Source: CAD feature listing. Evaluate the final solid. Frame: model axes, mm. A direction names the side the tool comes from. Coordinates: 2 decimals unless noted, no trailing zeros. Order: outer loops, then holes, each group sorted by start corner. A loop starts at its lowest first (then second) coordinate and runs counter-clockwise, first axis right, second up. Notation, with made-up numbers: (8.5, 30.25) -> (18.5, 30.25) arc R24 cw to (18.5, 58.25) -> close; hole circle Ø11 at (8, 72.5). An arc over 180 degrees is marked (long way). Write item = value, one per line. Start each with the question number.
Item 1: Contact query for flat-ended pins moving along their axis: pin 1 (1.5 mm diameter, centred on y = -428.5, z = 632, fed in from -X); pin 2 (1.5 mm diameter, centred on x = 108, y = -996.5, fed in from +Z); pin 3 (10 mm diameter, centred on x = 606, z = 1258, fed in from -Y). Output: stop coordinate, or through.
Item 2: Section query A-A (x = 641). Output: boundary loops of the cut face in (y, z).
Item 3: Section query B-B (y = -1621.5). Output: boundary loops of the cut face in (x, z), then the cut area to 3 significant figures.
Item 4: Section query D-D (x = 494.5). Output: boundary loops of the cut face in (y, z), then the cut area to 3 significant figures.
Item 5: Set-up query: faces 1 (the flat face through (351, -1102, 0)), 2 (the flat face through (509, -2033, 273.05)), 3 (the flat face through (272, -1796, 546.1)). Return all of +Z, -Z, +X, -X, +Y, -Y with unobstructed straight access to the full face (end or side cutting, diameter ignored); none if empty.
Item 6: Section query C-C (z = 621.5). Output: boundary loops of the cut face in (x, y), then the cut area to 3 significant figures.
Item 7: Ray query, line 1 along Z through (x, y) = (220, -876.5); line 2 along Z through (x, y) = (356, -1162); line 3 along Y through (x, z) = (382, 1186). Return the intervals inside material, ascending. Write a range as [from, to].
```python
from build123d import *

# Parameters (mm, degrees)
F0_W      = 711.2
F0_H      = 2235.2
F1_DEPTH  = 273.05
F3_DEPTH  = 273.05
F4_W      = 711.2
F4_H      = 1524
F5_DEPTH  = 273.05
F6_W      = 711.2
F6_H      = 1143
F7_DEPTH  = 273.05
F8_W      = 711.2
F8_H      = 762
F9_DEPTH  = 273.05
F10_W     = 711.2
F10_H     = 381
F11_DEPTH = 273.05


with BuildPart() as f1:
    # F0 (on Top) → F1 (new body)
    with BuildSketch(Plane.XY):
        with Locations((355.6, -1117.6)):
            Rectangle(F0_W, F0_H)
    extrude(amount=F1_DEPTH)

    # F2 (on face) → F3 (join)
    with BuildSketch(Plane.XY.offset(273.05)):
        Polygon((0, 0), (0, -2235.2), (711.2, -1524), (711.2, 0), align=None)
    extrude(amount=F3_DEPTH)

    # F4 (on face) → F5 (join)
    with BuildSketch(Plane.XY.offset(546.1)):
        with Locations((355.6, -762)):
            Rectangle(F4_W, F4_H)
    extrude(amount=F5_DEPTH)

    # F6 (on face) → F7 (join)
    with BuildSketch(Plane.XY.offset(819.15)):
        with Locations((355.6, -571.5)):
            Rectangle(F6_W, F6_H)
    extrude(amount=F7_DEPTH)

    # F8 (on face) → F9 (join)
    with BuildSketch(Plane.XY.offset(1092.2)):
        with Locations((355.6, -381)):
            Rectangle(F8_W, F8_H)
    extrude(amount=F9_DEPTH)

    # F10 (on face) → F11 (join)
    with BuildSketch(Plane.XY.offset(1365.25)):
        with Locations((355.6, -190.5)):
            Rectangle(F10_W, F10_H)
    extrude(amount=F11_DEPTH)


solid = f1.part
```
Computed:
q1.pin_1 = 0
q1.pin_2 = 1092.2
q1.pin_3 = -762
q2.outline = (-2235.2, 0) -> (0, 0) -> (0, 1638.3) -> (-381, 1638.3) -> (-381, 1365.25) -> (-762, 1365.25) -> (-762, 1092.2) -> (-1143, 1092.2) -> (-1143, 819.15) -> (-1524, 819.15) -> (-1524, 546.1) -> (-1594.2, 546.1) -> (-1594.2, 273.05) -> (-2235.2, 273.05) -> close
q3.outline = (0, 0) -> (711.2, 0) -> (711.2, 273.05) -> (613.7, 273.05) -> (613.7, 546.1) -> (0, 546.1) -> close
q3.area = 362,000 mm^2
q4.outline = (-2235.2, 0) -> (0, 0) -> (0, 1638.3) -> (-381, 1638.3) -> (-381, 1365.25) -> (-762, 1365.25) -> (-762, 1092.2) -> (-1143, 1092.2) -> (-1143, 819.15) -> (-1524, 819.15) -> (-1524, 546.1) -> (-1740.7, 546.1) -> (-1740.7, 273.05) -> (-2235.2, 273.05) -> close
q4.area = 2,130,000 mm^2
q5.face_1 = -Z, +X, -X, +Y, -Y
q5.face_2 = +Z, +X, -Y
q5.face_3 = +Z, +X, -X, -Y
q6.outline = (0, -1524) -> (711.2, -1524) -> (711.2, 0) -> (0, 0) -> close
q6.area = 1,080,000 mm^2
q7.line_1 = [0, 1092.2]
q7.line_2 = [0, 819.15]
q7.line_3 = [-762, 0]
